Source: CAD feature listing. Evaluate the final solid. Frame: model axes, mm. A direction names the side the tool comes from. Give positions to 0.01 mm unless a question says otherwise; leave off trailing zeros. Order: outer loops, then holes, each group sorted by start corner. A loop starts at its lowest first (then second) coordinate and runs counter-clockwise, first axis right, second up.
from build123d import *

# Parameters (mm, degrees)
SKETCH_1_W               = 120
SKETCH_1_H               = 79
EXTRUDE_1_DEPTH          = 5
SKETCH_2_R               = 3.1
CUT_EXTRUDE_1_DEPTH      = 2
SKETCH_3_R               = 1.5
CUT_EXTRUDE_2_DEPTH      = 72.897496479
PATTERN_LINEAR_1_COUNT   = 3
PATTERN_LINEAR_1_PITCH   = 30
MIRROR_2_COPY_1_SKETCH_R = 3.1
MIRROR_2_COPY_1_DEPTH    = 2
MIRROR_2_COPY_2_SKETCH_R = 3.1
MIRROR_2_COPY_2_DEPTH    = 2
MIRROR_2_COPY_3_SKETCH_R = 1.5
MIRROR_2_COPY_3_DEPTH    = 72.897496479
MIRROR_2_COPY_4_SKETCH_R = 1.5
MIRROR_2_COPY_4_DEPTH    = 72.897496479
CUT_EXTRUDE_3_DEPTH      = 1.5
CUT_EXTRUDE_4_DEPTH      = 72.920094549
SKETCH_7_R               = 1.5
CUT_EXTRUDE_6_DEPTH      = 5
SKETCH_9_R               = 1.6
SKETCH_9_R_2             = 1.5
CUT_EXTRUDE_7_DEPTH      = 73.008680032
SKETCH_11_W              = 10
SKETCH_11_H              = 15
CUT_EXTRUDE_8_DEPTH      = 73.008680032


with BuildPart() as part:
    # 草图1 → 凸台-拉伸1 (new body)
    with BuildSketch(Plane.XY):
        Rectangle(SKETCH_1_W, SKETCH_1_H)
    extrude(amount=EXTRUDE_1_DEPTH)

    # 草图2 → 切除-拉伸1 (cut)
    with BuildSketch(Plane(origin=(0, 0, 0), x_dir=(-1, 0, 0), z_dir=(0, 0, -1))):
        with Locations((-42.655984764, -33)):
            Circle(SKETCH_2_R)
        with Locations((-30.655984764, -33)):
            Circle(SKETCH_2_R)
    cut_extrude_1 = extrude(amount=-CUT_EXTRUDE_1_DEPTH, mode=Mode.SUBTRACT)

    # 草图3 → 切除-拉伸2 (cut, through all)
    with BuildSketch(Plane(origin=(0, 0, 2), x_dir=(-1, 0, 0), z_dir=(0, 0, -1))):
        with Locations((-42.655984764, -33)):
            Circle(SKETCH_3_R)
        with Locations((-30.655984764, -33)):
            Circle(SKETCH_3_R)
    cut_extrude_2 = extrude(amount=-CUT_EXTRUDE_2_DEPTH, mode=Mode.SUBTRACT)

    # 阵列(线性)1: 切除-拉伸1, 切除-拉伸2 ×3
    with Locations(*[(-i * PATTERN_LINEAR_1_PITCH, 0, 0) for i in range(1, PATTERN_LINEAR_1_COUNT)]):
        add(cut_extrude_1, mode=Mode.SUBTRACT)
        add(cut_extrude_2, mode=Mode.SUBTRACT)

    # 镜向2: 切除-拉伸1, 切除-拉伸2 across plane
    add(cut_extrude_1.mirror(Plane.ZX), mode=Mode.SUBTRACT)
    add(cut_extrude_2.mirror(Plane.ZX), mode=Mode.SUBTRACT)

    # 镜向2 copy 1 sketch → 镜向2 copy 1 (cut)
    with BuildSketch(Plane(origin=(-30, 0, 0), x_dir=(-1, 0, 0), z_dir=(0, 0, -1))):
        with Locations((-42.655984764, 33)):
            Circle(MIRROR_2_COPY_1_SKETCH_R)
        with Locations((-30.655984764, 33)):
            Circle(MIRROR_2_COPY_1_SKETCH_R)
    extrude(amount=-MIRROR_2_COPY_1_DEPTH, mode=Mode.SUBTRACT)

    # 镜向2 copy 2 sketch → 镜向2 copy 2 (cut)
    with BuildSketch(Plane(origin=(-60, 0, 0), x_dir=(-1, 0, 0), z_dir=(0, 0, -1))):
        with Locations((-42.655984764, 33)):
            Circle(MIRROR_2_COPY_2_SKETCH_R)
        with Locations((-30.655984764, 33)):
            Circle(MIRROR_2_COPY_2_SKETCH_R)
    extrude(amount=-MIRROR_2_COPY_2_DEPTH, mode=Mode.SUBTRACT)

    # 镜向2 copy 3 sketch → 镜向2 copy 3 (cut, through all)
    with BuildSketch(Plane(origin=(-30, 0, 2), x_dir=(-1, 0, 0), z_dir=(0, 0, -1))):
        with Locations((-42.655984764, 33)):
            Circle(MIRROR_2_COPY_3_SKETCH_R)
        with Locations((-30.655984764, 33)):
            Circle(MIRROR_2_COPY_3_SKETCH_R)
    extrude(amount=-MIRROR_2_COPY_3_DEPTH, mode=Mode.SUBTRACT)

    # 镜向2 copy 4 sketch → 镜向2 copy 4 (cut, through all)
    with BuildSketch(Plane(origin=(-60, 0, 2), x_dir=(-1, 0, 0), z_dir=(0, 0, -1))):
        with Locations((-42.655984764, 33)):
            Circle(MIRROR_2_COPY_4_SKETCH_R)
        with Locations((-30.655984764, 33)):
            Circle(MIRROR_2_COPY_4_SKETCH_R)
    extrude(amount=-MIRROR_2_COPY_4_DEPTH, mode=Mode.SUBTRACT)

    # 草图4 → 切除-拉伸3 (cut)
    with BuildSketch(Plane(origin=(0, 0, 0), x_dir=(-1, 0, 0), z_dir=(0, 0, -1))):
        with BuildLine():
            Line((34, 15.1), (54, 15.1))
            ThreePointArc((54, 15.1), (57.1, 12), (54, 8.9))
            Line((54, 8.9), (34, 8.9))
            ThreePointArc((34, 8.9), (30.9, 12), (34, 15.1))
        make_face()
        with BuildLine():
            Line((34, -21.1), (54, -21.1))
            ThreePointArc((54, -21.1), (57.1, -18), (54, -14.9))
            Line((54, -14.9), (34, -14.9))
            ThreePointArc((34, -14.9), (30.9, -18), (34, -21.1))
        make_face()
    extrude(amount=-CUT_EXTRUDE_3_DEPTH, mode=Mode.SUBTRACT)

    # 草图5 → 切除-拉伸4 (cut, through all)
    with BuildSketch(Plane(origin=(0, 0, 1.5), x_dir=(-1, 0, 0), z_dir=(0, 0, -1))):
        with BuildLine():
            Line((54, 10.5), (34, 10.5))
            ThreePointArc((34, 10.5), (32.5, 12), (34, 13.5))
            Line((34, 13.5), (54, 13.5))
            ThreePointArc((54, 13.5), (55.5, 12), (54, 10.5))
        make_face()
        with BuildLine():
            Line((54, -16.5), (34, -16.5))
            ThreePointArc((34, -16.5), (32.5, -18), (34, -19.5))
            Line((34, -19.5), (54, -19.5))
            ThreePointArc((54, -19.5), (55.5, -18), (54, -16.5))
        make_face()
    extrude(amount=-CUT_EXTRUDE_4_DEPTH, mode=Mode.SUBTRACT)

    # 草图7 → 切除-拉伸6 (cut)
    with BuildSketch(Plane.XZ.offset(39.5)):
        with Locations(Location((51.655984764, 2.5, 0), (0, 0, 270))):
            Circle(SKETCH_7_R)
        with Locations(Location((21.655984764, 2.5, 0), (0, 0, 270))):
            Circle(SKETCH_7_R)
        with Locations(Location((-8.344015236, 2.5, 0), (0, 0, 270))):
            Circle(SKETCH_7_R)
        with Locations(Location((-38.344015236, 2.5, 0), (0, 0, 270))):
            Circle(SKETCH_7_R)
        with Locations(Location((-53.344015236, 2.5, 0), (0, 0, 270))):
            Circle(SKETCH_7_R)
    cut_extrude_6 = extrude(amount=-CUT_EXTRUDE_6_DEPTH, mode=Mode.SUBTRACT)

    # 镜向3: 切除-拉伸6 across plane
    add(cut_extrude_6.mirror(Plane.ZX), mode=Mode.SUBTRACT)

    # 草图9 → 切除-拉伸7 (cut, through all)
    with BuildSketch(Plane(origin=(0, 0, 0), x_dir=(-1, 0, 0), z_dir=(0, 0, -1))):
        with Locations((24.027682272, -28)):
            Circle(SKETCH_9_R)
        with Locations((34.027682272, -28)):
            Circle(SKETCH_9_R)
        with Locations((24.027682272, 28)):
            Circle(SKETCH_9_R)
        with Locations((34.027682272, 28)):
            Circle(SKETCH_9_R)
        with Locations((-19.103783252, 30.4)):
            Circle(SKETCH_9_R_2)
        with Locations((-54.903783252, 30.4)):
            Circle(SKETCH_9_R_2)
        with Locations((-19.103783252, -30.4)):
            Circle(SKETCH_9_R_2)
        with Locations((-54.903783252, -30.4)):
            Circle(SKETCH_9_R_2)
        with BuildLine():
            Line((-49.452559424, -20.266203112), (-49.452559424, 19.733796888))
            ThreePointArc((-49.452559424, 19.733796888), (-46.952559424, 22.233796888), (-44.452559424, 19.733796888))
            Line((-44.452559424, 19.733796888), (-44.452559424, -20.266203112))
            ThreePointArc((-44.452559424, -20.266203112), (-46.952559424, -22.766203112), (-49.452559424, -20.266203112))
        make_face()
        with BuildLine():
            Line((-34.452559424, -20.266203112), (-34.452559424, 19.733796888))
            ThreePointArc((-34.452559424, 19.733796888), (-31.952559424, 22.233796888), (-29.452559424, 19.733796888))
            Line((-29.452559424, 19.733796888), (-29.452559424, -20.266203112))
            ThreePointArc((-29.452559424, -20.266203112), (-31.952559424, -22.766203112), (-34.452559424, -20.266203112))
        make_face()
        with BuildLine():
            Line((-19.452559424, -20.266203112), (-19.452559424, 19.733796888))
            ThreePointArc((-19.452559424, 19.733796888), (-16.952559424, 22.233796888), (-14.452559424, 19.733796888))
            Line((-14.452559424, 19.733796888), (-14.452559424, -20.266203112))
            ThreePointArc((-14.452559424, -20.266203112), (-16.952559424, -22.766203112), (-19.452559424, -20.266203112))
        make_face()
        with BuildLine():
            Line((-4.452559424, -20.266203112), (-4.452559424, 19.733796888))
            ThreePointArc((-4.452559424, 19.733796888), (-1.952559424, 22.233796888), (0.547440576, 19.733796888))
            Line((0.547440576, 19.733796888), (0.547440576, -20.266203112))
            ThreePointArc((0.547440576, -20.266203112), (-1.952559424, -22.766203112), (-4.452559424, -20.266203112))
        make_face()
        with BuildLine():
            Line((10.547440576, -20.266203112), (10.547440576, 19.733796888))
            ThreePointArc((10.547440576, 19.733796888), (13.047440576, 22.233796888), (15.547440576, 19.733796888))
            Line((15.547440576, 19.733796888), (15.547440576, -20.266203112))
            ThreePointArc((15.547440576, -20.266203112), (13.047440576, -22.766203112), (10.547440576, -20.266203112))
        make_face()
    extrude(amount=-CUT_EXTRUDE_7_DEPTH, mode=Mode.SUBTRACT)

    # 草图11 → 切除-拉伸8 (cut, through all)
    with BuildSketch(Plane.XY.offset(5)):
        with Locations((-24.027682272, -3)):
            Rectangle(SKETCH_11_W, SKETCH_11_H)
        with Locations((-34.027682272, -3)):
            Rectangle(SKETCH_11_W, SKETCH_11_H)
    extrude(amount=-CUT_EXTRUDE_8_DEPTH, mode=Mode.SUBTRACT)


solid = part.part
(1) Access query for faces 1 (the cylindrical face through (10.989, -30.386, 0.986)), 2 (the flat face through (-53, 34.5, 3)), 3 (the flat face through (19.453, -1, 2)). Directions: +Z, -Z, +X, -X, +Y, -Y. A direction counts if a zero-diameter tool reaches every point of the face in a straight line with its end or side. Return the directions, or none.
(2) Section A-A, the plane y = -5.5. Return loops of the section in (x, z), plus the area to 3 significant figures.
(3) Draft query along Z for faces 4 (the flat face through (-8, -34.5, 3)), 5 (the cylindrical face through (32.155, -32.934, 3.479)), 6 (the flat face through (11, -32, 2)). Return one class per face: +Z half, -Z half, draft (parallel to the pull), parting line (faces both ways), or undercut.
(4) Pin query (flat end, axial travel): pin 1 Ø1.9 at (x, y) = (30, -32.5) entering from -Z; pin 2 Ø1.5 at (x, z) = (-38.5, 2.5) entering from +Y; pin 3 Ø1.5 at (x, z) = (51, 2.5) entering from -Y. Return the tip coordinate at first contact, or that it passes through.
(5) Section B-B, the plane y = -18. Count the separate pieces of the cut face and the enclosed holes in it, plus the area to 3 significant figures.
(6) Line query: line 1 along Y through (x, z) = (-54, 0.65); line 2 along X through (y, z) = (-36.5, 2.5); line 3 along Y through (x, z) = (-41.5, 4.75). Output: solid intervals per line, ascending.
Checks:
1. face 1: -Z
1. face 2: +Y
1. face 3: +Z, -Z
2. outline: (-60, 0) - (-39.03, 0) - (-39.03, 5) - (-60, 5) - close; (-19.03, 0) - (-15.55, 0) - (-15.55, 5) - (-19.03, 5) - close; (-10.55, 0) - (-0.55, 0) - (-0.55, 5) - (-10.55, 5) - close; (4.45, 0) - (14.45, 0) - (14.45, 5) - (4.45, 5) - close; (19.45, 0) - (29.45, 0) - (29.45, 5) - (19.45, 5) - close; (34.45, 0) - (44.45, 0) - (44.45, 5) - (34.45, 5) - close; (49.45, 0) - (60, 0) - (60, 5) - (49.45, 5) - close
2. area: 375 mm2
3. face 4: undercut
3. face 5: draft
3. face 6: -Z half
4. pin 1: stops at z = 2
4. pin 2: stops at y = 34.5
4. pin 3: stops at y = -34.5
5. separate pieces: 7
5. enclosed holes: 0
5. area: 355 mm2
6. line 1: y = -39.5 to -21.1, -14.9 to 8.9, 15.1 to 39.5
6. line 2: x = -60 to -54.84, -51.84 to -39.84, -36.84 to -9.84, -6.84 to 20.16, 23.16 to 50.16, 53.16 to 60
6. line 3: y = -39.5 to -19.5, -16.5 to 10.5, 13.5 to 39.5
